Design review of the part shown in the three views and the two pictorial views. Dimensions are in mm from the part's minimum x, y and z. A direction names the side the tool comes from. Coordinates: 2 decimals unless noted, no trailing zeros. Loops run counter-clockwise (first coordinate to the right, second up) from the corner with the lowest first, then second, coordinate; pieces in that order, holes last. Notation, with made-up numbers: (-16.75, 17.5) - (-5.75, 17.5) arc R23 ccw to (-5.75, 37.5) - close; hole circle Ø1 at (-16, 78). An arc over 180 degrees is marked (long way). One line per item, written item: value. Start each with the question number.
1. Take a section at C-C, the plane z = 37. State the section outline as (x, y) points.
2. Take a section at B-B, the plane x = 68.5. State the section outline as (y, z) points.
3. Take a section at D-D, the plane x = 36. State the section outline as (y, z) points (1 decimal), and give its area (3 significant figures).
4. Take a section at A-A, the plane z = 54. State the section outline as (x, y) points.
5. To check wall thickness, follow line 1 (Z direction, x = 41, y = 4.75); line 2 (Z direction, x = 20.5, y = 6.25); line 3 (Z direction, x = 38.5, y = 6.75) (1 decimal). State the ranges of each line that lie inside material, in increasing order. Write a range as from..to.
6. Insertion check: pin 1 (8 mm diameter, centred on x = 55.5, z = 28.5, fed in from +Y); pin 2 (2 mm diameter, centred on y = 7, z = 8.5, fed in from -X); pin 3 (0.8 mm diameter, centred on y = 1.5, z = 49.5, fed in from +X) (1 decimal); pin 4 (4.5 mm diameter, centred on x = 69, y = 4.5, fed in from -Z). Each pin has a flat end and moves straight along its axis. Give the tip position at first contact, or say it passes through.
7. For the marked faces 1, 2 and 3, list the 3-axis set-ups (+Z, -Z, +X, -X, +Y, -Y) from which the entire face can be reached by the end or side of a thin tool; tool diameter is ignored.
8. The part is to be moulded in two halves that separate along X. For the marked faces 4, 5, 6 and 7, say which applies: released by +X, released by -X, zero draft, split by the parting line, or undercut.
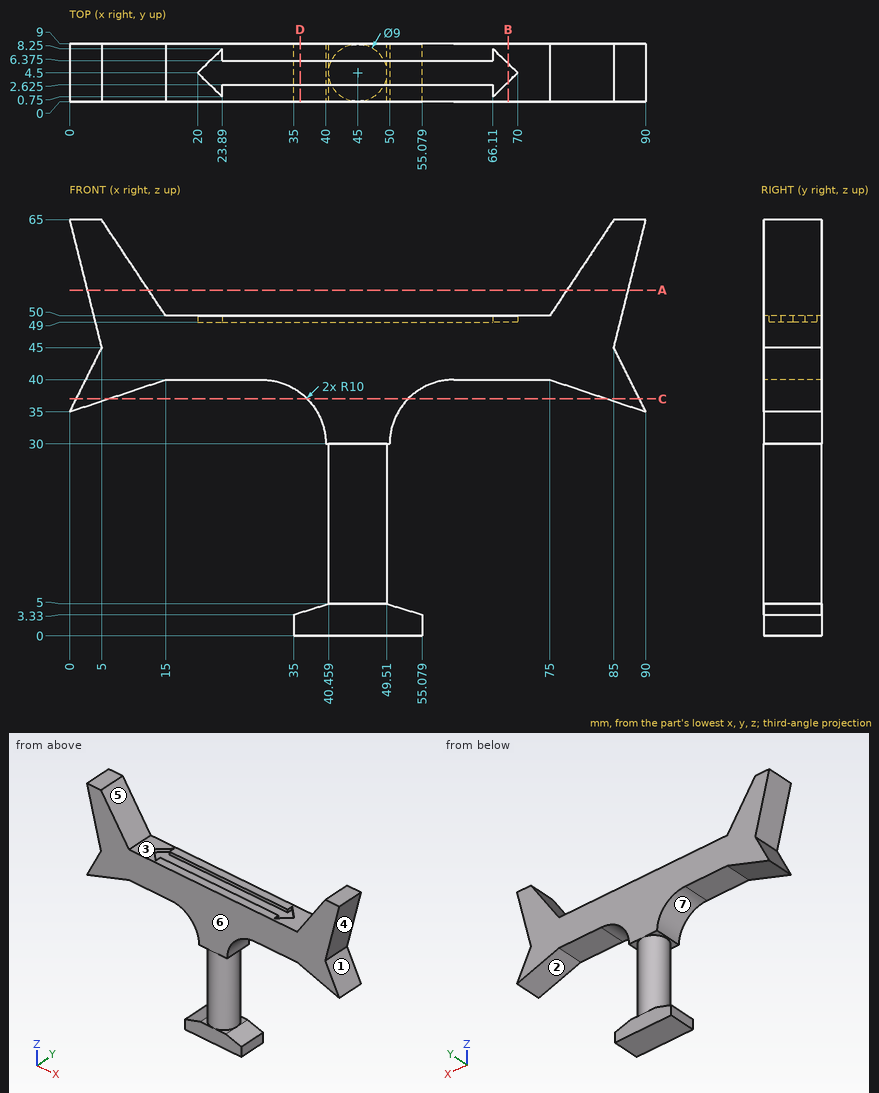
Solutions:
1. outline: (1, 0) - (6, 0) - (6, 9) - (1, 9) - close; (37.14, 0) - (52.86, 0) - (52.86, 9) - (37.14, 9) - close; (84, 0) - (89, 0) - (89, 9) - (84, 9) - close
2. outline: (0, 40) - (9, 40) - (9, 50) - (5.95, 50) - (5.95, 49) - (3.05, 49) - (3.05, 50) - (0, 50) - close
3. outline: (0, 0) - (9, 0) - (9, 3.6) - (0, 3.6) - close; (0, 38) - (9, 38) - (9, 50) - (6.4, 50) - (6.4, 49) - (2.6, 49) - (2.6, 50) - (0, 50) - close
3. area: 137 mm2
4. outline: (2.75, 0) - (12.33, 0) - (12.33, 9) - (2.75, 9) - close; (77.67, 0) - (87.25, 0) - (87.25, 9) - (77.67, 9) - close
5. line 1: 0..49
5. line 2: 40..50
5. line 3: 0..4.4, 35.3..50
6. pin 1: through
6. pin 2: x = 40.76
6. pin 3: x = 86.2
6. pin 4: z = 40
7. face 1: +X, +Y, -Y
7. face 2: -Z, +Y, -Y
7. face 3: +Z, +Y, -Y
8. face 4: released by +X
8. face 5: undercut
8. face 6: zero draft
8. face 7: undercut
